Verification items for the finished model (mm, model axes). Face numbers are marked on the shaded views. A direction names the side the tool comes from. Give positions to 0.01 mm unless a question says otherwise; leave off trailing zeros. Order: outer loops, then holes, each group sorted by start corner. A loop starts at its lowest first (then second) coordinate and runs counter-clockwise, first axis right, second up.
(1) Sectioned sample at C-C on z = 1.95. Record the cut outline in (x, y) (3 decimals).
(2) Sectioned sample at A-A on y = 0. Record the cut outline in (x, z), plus the area to 3 significant figures.
(3) Scan lines: L1, parallel to Y at x = -1.25, z = 1.7 (3 decimals); L2, parallel to Y at x = 2.75, z = 0.3; L3, parallel to X at y = -0.5, z = 3.55. Record each from-to range of solid material in increasing order.
(4) Access from +Z, -Z, +X, -X, +Y, -Y to the whole of each face (thin tool, end or side, straight path). Record for the marked faces 5 and 6.
(5) Gauge pin test, flat ends, axial feed: pin 1 (0.7 mm diameter, centred on x = 1.5, z = 3, fed in from -Y); pin 2 (0.7 mm diameter, centred on y = 1.5, z = 2, fed in from -X); pin 3 (1 mm diameter, centred on x = 2, z = 1.5, fed in from +Y). Record the tip position at first contact, or that the pin passes through.
(6) Mould release check, pull along X, two halves, no side actions. Record for the marked faces 1, 2, 3 and 4: pulls with the +X half, pulls with the -X half, needs draft (parallel to the pull), parting line crosses it, or undercut.
```python
from build123d import *

# Parameters (mm, degrees)
ESQUISSE1_R        = 3.25
BOSS_EXTRU_1_DEPTH = 6


with BuildPart() as part:
    # Esquisse1 → Boss.-Extru.1 (new body)
    with BuildSketch(Plane.XY):
        Circle(ESQUISSE1_R)
        with BuildLine():
            Line((2.125, -0.725), (1.197653957, -0.725))
            ThreePointArc((1.197653957, -0.725), (0.989949494, -0.989949494), (0.725, -1.197653957))
            Line((0.725, -1.197653957), (0.725, -2.125))
            ThreePointArc((0.725, -2.125), (0, -2.85), (-0.725, -2.125))
            Line((-0.725, -2.125), (-0.725, -1.197653957))
            ThreePointArc((-0.725, -1.197653957), (-0.989949494, -0.989949494), (-1.197653957, -0.725))
            Line((-1.197653957, -0.725), (-2.125, -0.725))
            ThreePointArc((-2.125, -0.725), (-2.85, 0), (-2.125, 0.725))
            Line((-2.125, 0.725), (-1.197653957, 0.725))
            ThreePointArc((-1.197653957, 0.725), (-0.989949494, 0.989949494), (-0.725, 1.197653957))
            Line((-0.725, 1.197653957), (-0.725, 2.125))
            ThreePointArc((-0.725, 2.125), (0, 2.85), (0.725, 2.125))
            Line((0.725, 2.125), (0.725, 1.197653957))
            ThreePointArc((0.725, 1.197653957), (0.989949494, 0.989949494), (1.197653957, 0.725))
            Line((1.197653957, 0.725), (2.125, 0.725))
            ThreePointArc((2.125, 0.725), (2.85, 0), (2.125, -0.725))
        make_face(mode=Mode.SUBTRACT)
    extrude(amount=BOSS_EXTRU_1_DEPTH)


solid = part.part
```
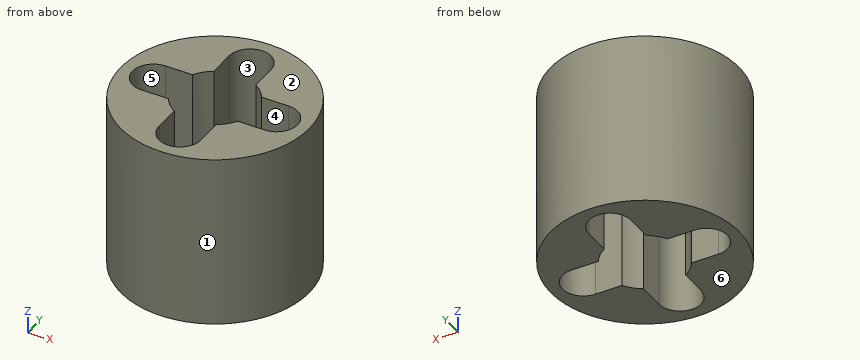
Ans:
1. outline: circle Ø6.5 at (0, 0); hole (-2.125, -0.725) - (-1.198, -0.725) arc R1.4 ccw to (-0.725, -1.198) - (-0.725, -2.125) arc R0.725 ccw to (0.725, -2.125) - (0.725, -1.198) arc R1.4 ccw to (1.198, -0.725) - (2.125, -0.725) arc R0.725 ccw to (2.125, 0.725) - (1.198, 0.725) arc R1.4 ccw to (0.725, 1.198) - (0.725, 2.125) arc R0.725 ccw to (-0.725, 2.125) - (-0.725, 1.198) arc R1.4 ccw to (-1.198, 0.725) - (-2.125, 0.725) arc R0.725 ccw to start
2. outline: (-3.25, 0) - (-2.85, 0) - (-2.85, 6) - (-3.25, 6) - close; (2.85, 0) - (3.25, 0) - (3.25, 6) - (2.85, 6) - close
2. area: 4.80 mm2
3. L1: y = -3 to -0.725, 0.725 to 3
3. L2: y = -1.73 to -0.37, 0.37 to 1.73
3. L3: x = -3.21 to -2.65, 2.65 to 3.21
4. face 5: +Z, -Z
4. face 6: -Z, +X, -X, +Y, -Y
5. pin 1: stops at y = -3.04
5. pin 2: stops at x = -3.04
5. pin 3: stops at y = 2.88
6. face 1: parting line crosses it
6. face 2: needs draft
6. face 3: undercut
6. face 4: undercut
